```python
from build123d import *


with BuildPart() as f1:
    # F0 (on Front) → F1 (revolve)
    with BuildSketch(Plane.XZ):
        with BuildLine():
            Line((0, -55), (0, 5))
            ThreePointArc((0, 5), (-3.535534, 3.535534), (-5, 0))
            Line((-5, 0), (-5, -1.918864))
            Line((-5, -1.918864), (-4.511429, -1.918864))
            Line((-4.511429, -1.918864), (-4.511429, -3.918864))
            Line((-4.511429, -3.918864), (-5, -3.918864))
            Line((-5, -3.918864), (-5, -5.237238))
            Line((-5, -5.237238), (-4.511429, -5.237238))
            Line((-4.511429, -5.237238), (-4.511429, -7.237238))
            Line((-4.511429, -7.237238), (-5, -7.237238))
            Line((-5, -7.237238), (-5, -55))
            Line((-5, -55), (0, -55))
        make_face()
    revolve(axis=Axis((0, 0, -25), (0, 0, 1)))


solid = f1.part
```
Input: part model. Units: mm. Frame: model coordinates. A direction names the side the tool comes from. Round coordinates to 2 decimals unless told otherwise and drop trailing zeros. Write each loop counter-clockwise with the first axis right and the second up, starting at its lowest first coordinate (ties: lowest second). Pieces come first, ordered by that corner, then holes. Notation, with made-up numbers: (30.25, 32.25) - (83.25, 32.25) arc R28 ccw to (83.25, 55.25) - close; hole circle Ø9 at (51.25, 48). An arc over 180 degrees is marked (long way). Write item = value, one per line.
(1) Access query for faces 1 (the cylindrical face through (1, 4.4, -2.9)), 2 (the cylindrical face through (1.08, 4.88, -4.59)). Directions: +Z, -Z, +X, -X, +Y, -Y. A direction counts if a zero-diameter tool reaches every point of the face in a straight line with its end or side. Return the directions, or none.
Geometry check:
face_1 = none
face_2 = +Z, -Z
(2) Material intervals for probe 1 along Y at (x, z) = (0.25, -38); probe 2 along Z at (x, y) = (4, -1.75); probe 3 along Z at (x, y) = (-2.75, 0.5), sorted ascending.
Geometry check:
probe_1 = -4.99 to 4.99
probe_2 = -55 to 2.44
probe_3 = -55 to 4.15
(3) Pull-direction query (Z, two-part tool) for faces 3 (the cylindrical face through (1, 4.4, -6.3)), 4 (the flat face through (0, 0, -55)), 5 (the cylindrical face through (1.08, 4.88, -0.97)); classes: +Z half, -Z half, draft (parallel to the pull), parting line (faces both ways), or undercut.
Geometry check:
face_3 = undercut
face_4 = -Z half
face_5 = draft
(4) Section query A-A on z = -34.5. Output: boundary loops of the cut face in (x, y), then the cut area to 3 significant figures.
Geometry check:
outline = circle Ø10 at (0, 0)
area = 78.5 mm^2
(5) Contact query for flat-ended pins moving along their axis: pin 1 Ø2 at (x, y) = (-1, -1.5) entering from +Z; pin 2 Ø3 at (x, z) = (-3.5, -8.5) entering from -Y; pin 3 Ø1.5 at (x, y) = (2, 3) entering from +Z. Output: stop coordinate, or through.
Geometry check:
pin_1 = 4.94
pin_2 = -4.58
pin_3 = 4.1
